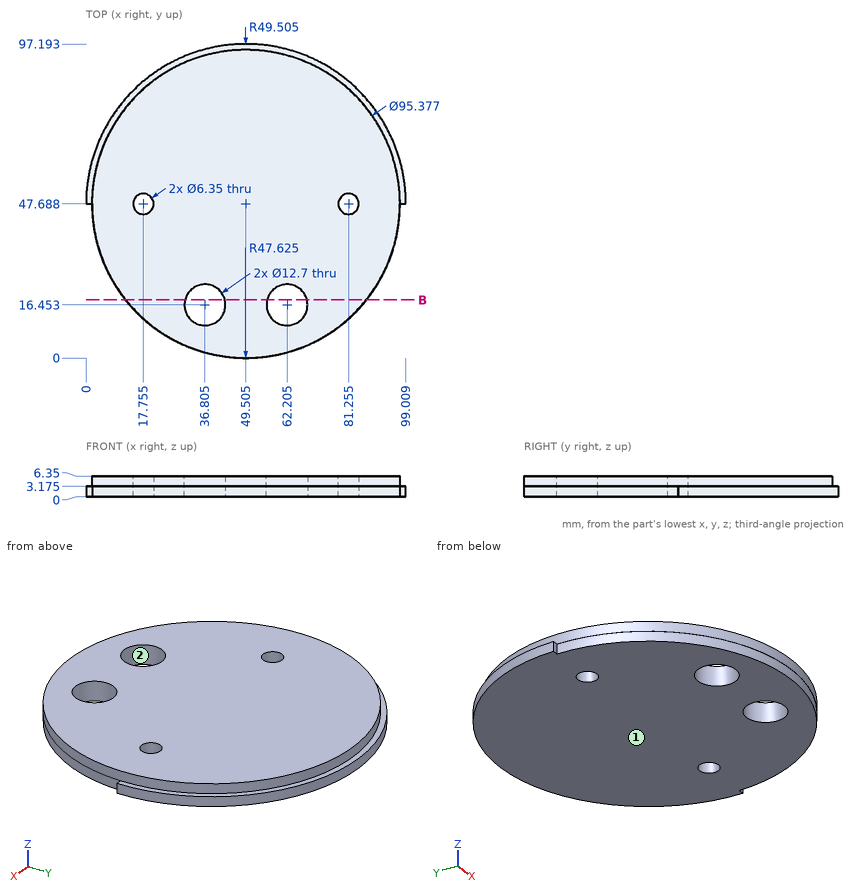
Here's the drawing with two shaded views (mm, measured from the low corner). I have some questions. Coordinates: 2 decimals unless noted, no trailing zeros. Answer in a Markdown table with one row per item.
(1) Will these pins go through, and if not, where does the flat tip stop? pin 1 Ø1.5 at (y, z) = (18, 5.5) entering from +X; pin 2 Ø0.9 at (x, z) = (98.5, 1.5) entering from -Y; pin 3 Ø3 at (y, z) = (53.5, 2.5) entering from +X; pin 4 Ø10 at (x, y) = (36.8, 16.45) entering from -Z.
Results found:
| item | result |
|---|---|
| pin 1 | stops at x = 87.41 |
| pin 2 | stops at y = 47.69 |
| pin 3 | stops at x = 98.82 |
| pin 4 | passes through |
(2) Thinking about a two-plate mould opening in X: for the marked faces 1 and 2, which applies, released by +X, released by -X, zero draft, split by the parting line, or undercut?
Results found:
| item | result |
|---|---|
| face 1 | zero draft |
| face 2 | undercut |
(3) Imagine slicing it at B-B (y = 18). Give the number of separate pieces and of enclosed holes in the cut face, plus the area to 3 significant figures.
Results found:
| item | result |
|---|---|
| separate pieces | 3 |
| enclosed holes | 0 |
| area | 317 mm^2 |
(4) If I drill on probe 1 along Y at (x, z) = (42, 2) (1 decimal); probe 2 along X at (y, z) = (15.5, 0.5) (1 decimal); probe 3 along Y at (x, z) = (40, 1.5) (1 decimal), over which ranges is the centre line in solid material (lowest first)?
Results found:
| item | result |
|---|---|
| probe 1 | y = 0.7 to 12.8, 20.1 to 96.6 |
| probe 2 | x = 14.4 to 30.5, 43.1 to 55.9, 68.5 to 84.6 |
| probe 3 | y = 1 to 11, 21.9 to 96.3 |
